from build123d import *

# Parameters (mm, degrees)
SKETCH2_W              = 60
SKETCH2_H              = 60
BOSS_EXTRUDE1_DEPTH    = 5
SKETCH3_W              = 60
SKETCH3_H              = 5
BOSS_EXTRUDE2_DEPTH    = 60
CUT_EXTRUDE1_REACH     = 106.163
SKETCH4_R              = 11.5
CUT_EXTRUDE2_REACH     = 105.923
CONVERT_SOLID1_DEPTH   = 60
CONVERT_SOLID1_2_DEPTH = 60
FILLET1_R              = 10
FILLET2_R              = 10
FILLET3_R              = 10
FILLET4_R              = 10


# Read off the part's stored shape, not the designer's step: Convert-Solid1
with BuildPart() as part:
    # Sketch2 → Boss-Extrude1 (new body)
    with BuildSketch(Plane.XY):
        with Locations((30, 30)):
            Rectangle(SKETCH2_W, SKETCH2_H)
    extrude(amount=BOSS_EXTRUDE1_DEPTH)

    # Sketch3 → Boss-Extrude2 (add)
    with BuildSketch(Plane.XY.offset(5)):
        with Locations((30, 57.5)):
            Rectangle(SKETCH3_W, SKETCH3_H)
    extrude(amount=BOSS_EXTRUDE2_DEPTH)

    # Sketch4 → Cut-Extrude1 (cut, up to next)
    with BuildSketch(Plane.XZ.offset(-55), mode=Mode.PRIVATE) as cut_extrude1_sk1:
        with Locations(Location((30, 42.5, 0), (0, 0, 270))):
            Circle(SKETCH4_R)
    cut_extrude1_tool1 = extrude(cut_extrude1_sk1.sketch, amount=-CUT_EXTRUDE1_REACH, mode=Mode.PRIVATE) & part.part
    add(cut_extrude1_tool1.solids().sort_by_distance((30, 55, 42.5))[0], mode=Mode.SUBTRACT)

    # Sketch5 → Cut-Extrude2 (cut, up to next)
    with BuildSketch(Plane.XY.offset(5), mode=Mode.PRIVATE) as cut_extrude2_sk1:
        with BuildLine():
            Line((15, 38.341687605), (15, 11.658312395))
            ThreePointArc((15, 11.658312395), (17.5, 7), (20, 11.658312395))
            Line((20, 11.658312395), (20, 38.341687605))
            ThreePointArc((20, 38.341687605), (17.5, 43), (15, 38.341687605))
        make_face()
    cut_extrude2_tool1 = extrude(cut_extrude2_sk1.sketch, amount=-CUT_EXTRUDE2_REACH, mode=Mode.PRIVATE) & part.part
    # Sketch5 → Cut-Extrude2 (cut, up to next)
    with BuildSketch(Plane.XY.offset(5), mode=Mode.PRIVATE) as cut_extrude2_sk2:
        with BuildLine():
            Line((40, 38.341687605), (40, 11.658312395))
            ThreePointArc((40, 11.658312395), (42.5, 7), (45, 11.658312395))
            Line((45, 11.658312395), (45, 38.341687605))
            ThreePointArc((45, 38.341687605), (42.5, 43), (40, 38.341687605))
        make_face()
    cut_extrude2_tool2 = extrude(cut_extrude2_sk2.sketch, amount=-CUT_EXTRUDE2_REACH, mode=Mode.PRIVATE) & part.part
    add(cut_extrude2_tool1.solids().sort_by_distance((17.5, 25, 5))[0], mode=Mode.SUBTRACT)
    add(cut_extrude2_tool2.solids().sort_by_distance((42.5, 25, 5))[0], mode=Mode.SUBTRACT)

    # Convert-Solid1 outline → Convert-Solid1 (cut)
    with BuildSketch(Plane.YZ):
        with BuildLine():
            Line((60, 65), (57.5, 65))
            Line((57.5, 65), (57.5, 10))
            ThreePointArc((57.5, 10), (55.303300859, 4.696699141), (50, 2.5))
            Line((50, 2.5), (0, 2.5))
            Line((0, 2.5), (0, 0))
            Line((0, 0), (60, 0))
            Line((60, 0), (60, 65))
        make_face()
    extrude(amount=CONVERT_SOLID1_DEPTH, mode=Mode.SUBTRACT)

    # Convert-Solid1 2 outline → Convert-Solid1 2 (add)
    with BuildSketch(Plane.YZ):
        with BuildLine():
            Line((55, 5), (55, 10))
            ThreePointArc((55, 10), (53.535533906, 6.464466094), (50, 5))
            Line((50, 5), (55, 5))
        make_face()
    extrude(amount=CONVERT_SOLID1_2_DEPTH)

    # Fillet1
    fillet1_edges = [part.edges().sort_by_distance(p)[0] for p in [
        (60, 56.25, 65),
    ]]
    fillet(fillet1_edges, radius=FILLET1_R)

    # Fillet2
    fillet2_edges = [part.edges().sort_by_distance(p)[0] for p in [
        (0, 56.25, 65),
    ]]
    fillet(fillet2_edges, radius=FILLET2_R)

    # Fillet3
    fillet3_edges = [part.edges().sort_by_distance(p)[0] for p in [
        (0, 0, 3.75),
    ]]
    fillet(fillet3_edges, radius=FILLET3_R)

    # Fillet4
    fillet4_edges = [part.edges().sort_by_distance(p)[0] for p in [
        (60, 0, 3.75),
    ]]
    fillet(fillet4_edges, radius=FILLET4_R)


solid = part.part
Can you work these out from the model? Positions are in its coordinate system, mm. A direction names the side the tool comes from. Give positions to 0.01 mm unless a question says otherwise; leave off trailing zeros. Write each loop counter-clockwise with the first axis right and the second up, starting at its lowest first coordinate (ties: lowest second). Pieces come first, ordered by that corner, then holes. Notation, with made-up numbers: (-9.5, 1.5) -> (39.5, 1.5) arc R27 cw to (39.5, 36.5) -> close; hole circle Ø6 at (-23.75, 52). An arc over 180 degrees is marked (long way). Answer as a JSON object with one key per item and string values. Group by question number.
Item 1: I'm going to push flat-ended pins straight in: P1, Ø2, axis at x = 23, y = 44.5, coming from the +Z side; P2, Ø1.5, axis at x = 44, y = 35, coming from the +Z side; P3, Ø16.5, axis at x = 23.5, z = 36, coming from the -Y side. Where does each tip first touch, or does it pass through?
Item 2: Suppose I cut it at D-D (z = 16.5). Please give me the cut outline in (x, y).
Item 3: Suppose I cut it at A-A (x = 30). Please give me the cut outline in (y, z), plus the area to 3 significant figures.
Item 4: Please list where these lines run through material, in increasing order: line 1 (X direction, y = 10, z = 3.25); line 2 (Y direction, x = 6.5, z = 48); line 3 (Z direction, x = 54, y = 36). Write a range as [from, to].
Item 5: Suppose I cut it at C-C (x = 17.5). Please give me the cut outline in (y, z), plus the area to 3 significant figures.
Item 6: For faces 1 (the face through (15, 25, 4)), 2 (the face through (60, 57, 17)), 3 (the face through (30, 25, 5)), which set-ups out of +Z, -Z, +X, -X, +Y, -Y let a thin tool reach every point of the face, with its end or its side?
Item 7: We'd pull the mould along X, two halves only. Please class faces 4 (the face through (36, 57.5, 32)), 5 (the face through (0, 57, 17)), 6 (the face through (20, 25, 4)): +X half, -X half, draft (parallel to the pull), parting line (faces both ways), or undercut.
Item 8: Suppose I cut it at B-B (z = 42.5). Please give me the cut outline in (x, y), plus the area to 3 significant figures.
Findings:
{
 "1": {"P1": "stops at z = 5", "P2": "passes through", "P3": "stops at y = 55"},
 "2": {"outline": "(0, 55) -> (60, 55) -> (60, 57.5) -> (0, 57.5) -> close"},
 "3": {"outline": "(0, 2.5) -> (50, 2.5) arc R7.5 ccw to (57.5, 10) -> (57.5, 31) -> (55, 31) -> (55, 10) arc R5 cw to (50, 5) -> (0, 5) -> close; (55, 54) -> (57.5, 54) -> (57.5, 65) -> (55, 65) -> close", "area": "230 mm²"},
 "4": {"line 1": "x = [0, 14.5], [20.5, 39.5], [45.5, 60]", "line 2": "y = [55, 57.5]", "line 3": "z = [2.5, 5]"},
 "5": {"outline": "(0, 2.5) -> (7, 2.5) -> (7, 5) -> (0, 5) -> close; (43, 2.5) -> (50, 2.5) arc R7.5 ccw to (57.5, 10) -> (57.5, 65) -> (55, 65) -> (55, 10) arc R5 cw to (50, 5) -> (43, 5) -> close", "area": "197 mm²"},
 "6": {"face 1": "+Z, -Z", "face 2": "+Z, -Z, +X, +Y, -Y", "face 3": "+Z, +X, -X, -Y"},
 "7": {"face 4": "draft", "face 5": "-X half", "face 6": "undercut"},
 "8": {"outline": "(0, 55) -> (18.5, 55) -> (18.5, 57.5) -> (0, 57.5) -> close; (41.5, 55) -> (60, 55) -> (60, 57.5) -> (41.5, 57.5) -> close", "area": "92.5 mm²"}
}
